from build123d import *

# Parameters (mm, degrees)
BOSS_EXTRU_1_DEPTH      = 30
ENL_V_MAT_EXTRU_1_REACH = 38.469
ESQUISSE2_R             = 3.5
ENL_V_MAT_EXTRU_2_REACH = 38.469
ESQUISSE3_R             = 1.75
ENL_V_MAT_EXTRU_3_REACH = 39.921
ESQUISSE4_W             = 5
ESQUISSE4_H             = 2


with BuildPart() as part:
    # Esquisse1 → Boss.-Extru.1 (new body)
    with BuildSketch(Plane.XY):
        Polygon((0, 0), (-19, 0), (0, 13.303943226), align=None)
    extrude(amount=BOSS_EXTRU_1_DEPTH)

    # Enlèv. mat.-Extru.1: up to this plane
    enl_v_mat_extru_1_end = Plane(origin=(-19, 0, 30), z_dir=(0.5735764363510416, -0.8191520442889949, 0))
    # Esquisse2 → Enlèv. mat.-Extru.1 (cut, up to the surface)
    with BuildSketch(Plane(origin=(0, 5, 0), x_dir=(-1, 0, 0), z_dir=(0, -1, 0)), mode=Mode.PRIVATE) as enl_v_mat_extru_1_sk1:
        with Locations(Location((7.5, -7.5, 0), (0, 0, 180))):
            Circle(ESQUISSE2_R)
    enl_v_mat_extru_1_tool1 = split(extrude(enl_v_mat_extru_1_sk1.sketch, amount=-ENL_V_MAT_EXTRU_1_REACH, mode=Mode.PRIVATE), bisect_by=enl_v_mat_extru_1_end, keep=Keep.BOTH, mode=Mode.PRIVATE)
    add(enl_v_mat_extru_1_tool1.solids().sort_by_distance((-7.5, 5, 7.5))[0], mode=Mode.SUBTRACT)
    # Esquisse2 → Enlèv. mat.-Extru.1 (cut, up to the surface)
    with BuildSketch(Plane(origin=(0, 5, 0), x_dir=(-1, 0, 0), z_dir=(0, -1, 0)), mode=Mode.PRIVATE) as enl_v_mat_extru_1_sk2:
        with Locations(Location((7.5, -22.5, 0), (0, 0, 180))):
            Circle(ESQUISSE2_R)
    enl_v_mat_extru_1_tool2 = split(extrude(enl_v_mat_extru_1_sk2.sketch, amount=-ENL_V_MAT_EXTRU_1_REACH, mode=Mode.PRIVATE), bisect_by=enl_v_mat_extru_1_end, keep=Keep.BOTH, mode=Mode.PRIVATE)
    add(enl_v_mat_extru_1_tool2.solids().sort_by_distance((-7.5, 5, 22.5))[0], mode=Mode.SUBTRACT)

    # Esquisse3 → Enlèv. mat.-Extru.2 (cut, up to next)
    with BuildSketch(Plane(origin=(0, 5, 0), x_dir=(1, 0, 0), z_dir=(0, 1, 0)), mode=Mode.PRIVATE) as enl_v_mat_extru_2_sk1:
        with Locations(Location((-7.5, -22.5, 0), (0, 0, 180))):
            Circle(ESQUISSE3_R)
    enl_v_mat_extru_2_tool1 = extrude(enl_v_mat_extru_2_sk1.sketch, amount=-ENL_V_MAT_EXTRU_2_REACH, mode=Mode.PRIVATE) & part.part
    # Esquisse3 → Enlèv. mat.-Extru.2 (cut, up to next)
    with BuildSketch(Plane(origin=(0, 5, 0), x_dir=(1, 0, 0), z_dir=(0, 1, 0)), mode=Mode.PRIVATE) as enl_v_mat_extru_2_sk2:
        with Locations(Location((-7.5, -7.5, 0), (0, 0, 180))):
            Circle(ESQUISSE3_R)
    enl_v_mat_extru_2_tool2 = extrude(enl_v_mat_extru_2_sk2.sketch, amount=-ENL_V_MAT_EXTRU_2_REACH, mode=Mode.PRIVATE) & part.part
    add(enl_v_mat_extru_2_tool1.solids().sort_by_distance((-7.5, 5, 22.5))[0], mode=Mode.SUBTRACT)
    add(enl_v_mat_extru_2_tool2.solids().sort_by_distance((-7.5, 5, 7.5))[0], mode=Mode.SUBTRACT)

    # Enlèv. mat.-Extru.3: up to this plane
    enl_v_mat_extru_3_end = Plane(origin=(-19, 0, 30), z_dir=(0.5735764363510416, -0.8191520442889949, 0))
    # Esquisse4 → Enlèv. mat.-Extru.3 (cut, up to the surface)
    with BuildSketch(Plane(origin=(0, 0, 0), x_dir=(0, 0, -1), z_dir=(1, 0, 0)), mode=Mode.PRIVATE) as enl_v_mat_extru_3_sk1:
        with Locations((-15, 1)):
            Rectangle(ESQUISSE4_W, ESQUISSE4_H)
    enl_v_mat_extru_3_tool1 = split(extrude(enl_v_mat_extru_3_sk1.sketch, amount=-ENL_V_MAT_EXTRU_3_REACH, mode=Mode.PRIVATE), bisect_by=enl_v_mat_extru_3_end, keep=Keep.BOTH, mode=Mode.PRIVATE)
    add(enl_v_mat_extru_3_tool1.solids().sort_by_distance((0, 1, 15))[0], mode=Mode.SUBTRACT)


solid = part.part
CAD build for the part. Positions are in the model's coordinates, mm. A direction names the side the tool comes from. Round coordinates to 2 decimals unless told otherwise and drop trailing zeros. Write each loop counter-clockwise with the first axis right and the second up, starting at its lowest first coordinate (ties: lowest second). Pieces come first, ordered by that corner, then holes. Notation, with made-up numbers: (82, 86) -> (130, 86) arc R7 cw to (130, 93) -> close; hole circle Ø2 at (-39.5, -12). An arc over 180 degrees is marked (long way). Answer as a JSON object with one key per item and string values.
(1) Which spindle directions (+Z, -Z, +X, -X, +Y, -Y) get a long thin tool onto all of the face, cutting with end or side? Do faces 1 (the face through (-9, 1, 12.5)), 2 (the face through (-4.16, 7.1, 8.55)), 3 (the face through (-9.63, 6.56, 14.79)). Say none if no direction does.
Reported:
{"face 1": "+X, -X, -Y", "face 2": "+Y", "face 3": "+Z, -Z, -X, +Y"}
(2) Band-saw the part on C-C, the plane x = -7.5. List the corners of the cut face in (y, z).
Reported:
{"outline": "(0, 0) -> (8.05, 0) -> (8.05, 4) -> (5, 4) -> (5, 5.75) -> (0, 5.75) -> close; (0, 9.25) -> (5, 9.25) -> (5, 11) -> (8.05, 11) -> (8.05, 19) -> (5, 19) -> (5, 20.75) -> (0, 20.75) -> (0, 17.5) -> (2, 17.5) -> (2, 12.5) -> (0, 12.5) -> close; (0, 24.25) -> (5, 24.25) -> (5, 26) -> (8.05, 26) -> (8.05, 30) -> (0, 30) -> close"}
(3) Band-saw the part on D-D, the plane z = 11.5. List the corners of the cut face in (x, y), then the cut area to 3 significant figures.
Reported:
{"outline": "(-19, 0) -> (0, 0) -> (0, 13.3) -> close", "area": "126 mm^2"}
(4) Two-plate mould, pull along Z, no slides. Class faces 4 (the face through (-9, 1, 17.5)), 5 (the face through (-9, 0, 6)), 6 (the face through (-5, 4, 0)): +Z half, -Z half, draft (parallel to the pull), parting line (faces both ways), or undercut.
Reported:
{"face 4": "undercut", "face 5": "draft", "face 6": "-Z half"}
(5) Pin check, flat tips, straight feed: P1, Ø4, axis at x = -7.5, z = 22.5, coming from the +Y side; P2, Ø7.5, axis at x = -8.5, z = 6, coming from the +Y side; P3, Ø4, axis at y = 5.5, z = 25.5, coming from the -X side; P4, Ø3, axis at x = -7.5, z = 7.5, coming from the +Y side. Stop position of each tip, or through.
Reported:
{"P1": "stops at y = 5", "P2": "stops at y = 9.92", "P3": "stops at x = -14", "P4": "passes through"}
(6) Band-saw the part on A-A, the plane z = 22.5. List the corners of the cut face in (x, y), then the cut area to 3 significant figures.
Reported:
{"outline": "(-19, 0) -> (-9.25, 0) -> (-9.25, 5) -> (-11, 5) -> (-11, 5.6) -> close; (-5.75, 0) -> (0, 0) -> (0, 13.3) -> (-4, 10.5) -> (-4, 5) -> (-5.75, 5) -> close", "area": "87.5 mm^2"}
(7) Band-saw the part on B-B, the plane x = -11.75. List the corners of the cut face in (y, z), then the cut area to 3 significant figures.
Reported:
{"outline": "(0, 0) -> (5.08, 0) -> (5.08, 30) -> (0, 30) -> (0, 17.5) -> (2, 17.5) -> (2, 12.5) -> (0, 12.5) -> close", "area": "142 mm^2"}
(8) Probe probe 1 along Z at (x, y) = (-7.5, 6.9); probe 2 along Z at (x, y) = (-6, 7.5); probe 3 along Y at (x, z) = (-6, 23.75). List the from-to ranges inside material, lowest first. Write a range as [from, to].
Reported:
{"probe 1": "z = [0, 4], [11, 19], [26, 30]", "probe 2": "z = [0, 4.34], [10.66, 19.34], [25.66, 30]", "probe 3": "y = [0, 5]"}
